The model under review builds one solid part; all positions refer to its coordinate system, in mm. Face numbers are marked on the shaded views. A direction names the side the tool comes from. Round coordinates to 2 decimals unless told otherwise and drop trailing zeros. Write each loop counter-clockwise with the first axis right and the second up, starting at its lowest first coordinate (ties: lowest second). Pieces come first, ordered by that corner, then holes. Notation, with made-up numbers: (-4, 88) -> (10, 88) arc R28 cw to (10, 126) -> close; hole circle Ø11 at (39, 4.5). An arc over 180 degrees is marked (long way). Answer as a JSON object with one key per item and string values. Group by question number.
1) Mouldability with a two-part tool opening along Z and no side actions: class the marked faces 1, 2 and 3 as pulls with the +Z half, pulls with the -Z half, needs draft (parallel to the pull), parting line crosses it, or undercut.
2) We need section D-D, the plane z = -7.75. Write out the cut boundary in (x, y), then the cut area to 3 significant figures.
3) We need section A-A, the plane x = 39.65. Write out the cut boundary in (y, z).
4) We need section B-B, the plane z = -3.5. Write out the cut boundary in (x, y), then the cut area to 3 significant figures.
5) We need section C-C, the plane y = 5.25. Write out the cut boundary in (x, z).
6) Insertion check: pin 1 Ø3.5 at (x, z) = (4.1, -7.75) entering from +Y. The pin has a flat end and moves straight along its axis. Give the tip position at first contact, or say it passes through.
7) Machinability: for the marked faces 4 and 5, which of the approach directions +Z, -Z, +X, -X, +Y, -Y give a long, thin tool a straight path to every point of the face, cutting with its end or side? Answer none if there is none.
8) To check wall thickness, follow probe 1 along X at (y, z) = (0.5, -7.75); probe 2 along X at (y, z) = (10, -11.75); probe 3 along X at (y, z) = (1.25, -3.5). State the ranges of each line that lie inside material, in increasing order. Write a range as [from, to].
from build123d import *

# Parameters (mm, degrees)
SKETCH_1_W          = 50
SKETCH_1_H          = 15.5
EXTRUDE_1_DEPTH     = 14
SKETCH_2_W          = 47
SKETCH_2_H          = 12.5
CUT_EXTRUDE_1_DEPTH = 12
SKETCH_4_R          = 1.15
SKETCH_4_R_2        = 1.806882298
SKETCH_4_W          = 23
SKETCH_4_H          = 12.5
CUT_EXTRUDE_2_DEPTH = 2


with BuildPart() as part:
    # 草图1 → 凸台-拉伸1 (new body)
    with BuildSketch(Plane(origin=(0, 0, 0), x_dir=(1, 0, 0), z_dir=(0, 1, 0))):
        with Locations((25, 7.75)):
            Rectangle(SKETCH_1_W, SKETCH_1_H)
    extrude(amount=EXTRUDE_1_DEPTH)

    # 草图2 → 切除-拉伸1 (cut)
    with BuildSketch(Plane(origin=(0, 14, 0), x_dir=(1, 0, 0), z_dir=(0, 1, 0))):
        with Locations((25, 7.75)):
            Rectangle(SKETCH_2_W, SKETCH_2_H)
    extrude(amount=-CUT_EXTRUDE_1_DEPTH, mode=Mode.SUBTRACT)

    # 草图4 → 切除-拉伸2 (cut)
    with BuildSketch(Plane(origin=(0, 2, 0), x_dir=(1, 0, 0), z_dir=(0, 1, 0))):
        with Locations(Location((4.1, 7.75, 0), (0, 0, 270))):
            Circle(SKETCH_4_R)
        with Locations(Location((31.9, 7.75, 0), (0, 0, 270))):
            Circle(SKETCH_4_R)
        with Locations(Location((39.65, 7.75, 0), (0, 0, 270))):
            Circle(SKETCH_4_R_2)
        with Locations((18, 7.75)):
            Rectangle(SKETCH_4_W, SKETCH_4_H)
    extrude(amount=-CUT_EXTRUDE_2_DEPTH, mode=Mode.SUBTRACT)


solid = part.part
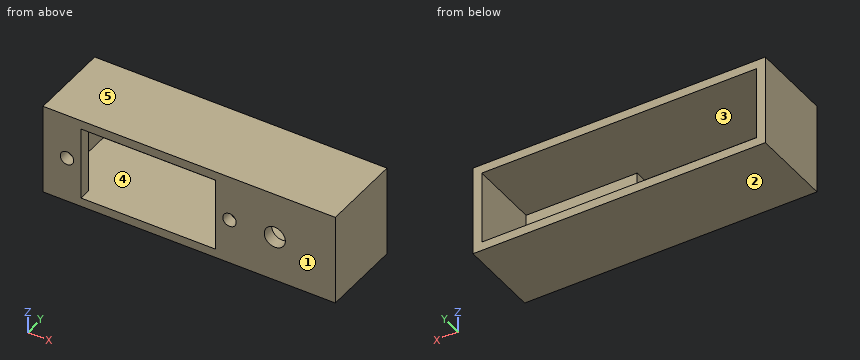
Here are the results:
{
 "1": {"face 1": "needs draft", "face 2": "pulls with the -Z half", "face 3": "undercut"},
 "2": {"outline": "(0, 0) -> (2.95, 0) -> (2.95, 2) -> (1.5, 2) -> (1.5, 14) -> (0, 14) -> close; (5.25, 0) -> (6.5, 0) -> (6.5, 2) -> (5.25, 2) -> close; (29.5, 0) -> (30.75, 0) -> (30.75, 2) -> (29.5, 2) -> close; (33.05, 0) -> (37.84, 0) -> (37.84, 2) -> (33.05, 2) -> close; (41.46, 0) -> (50, 0) -> (50, 14) -> (48.5, 14) -> (48.5, 2) -> (41.46, 2) -> close", "area": "73.6 mm^2"},
 "3": {"outline": "(0, -15.5) -> (14, -15.5) -> (14, -14) -> (2, -14) -> (2, -9.56) -> (0, -9.56) -> close; (0, -5.94) -> (2, -5.94) -> (2, -1.5) -> (14, -1.5) -> (14, 0) -> (0, 0) -> close"},
 "4": {"outline": "(0, 0) -> (6.5, 0) -> (6.5, 2) -> (1.5, 2) -> (1.5, 14) -> (0, 14) -> close; (29.5, 0) -> (50, 0) -> (50, 14) -> (48.5, 14) -> (48.5, 2) -> (29.5, 2) -> close", "area": "90.0 mm^2"},
 "5": {"outline": "(0, -15.5) -> (50, -15.5) -> (50, 0) -> (0, 0) -> close; hole (1.5, -14) -> (48.5, -14) -> (48.5, -1.5) -> (1.5, -1.5) -> close"},
 "6": {"pin 1": "stops at y = 2"},
 "7": {"face 4": "+Y", "face 5": "+Z, +X, -X, +Y, -Y"},
 "8": {"probe 1": "x = [0, 2.95], [5.25, 6.5], [29.5, 30.75], [33.05, 37.84], [41.46, 50]", "probe 2": "x = [0, 1.5], [48.5, 50]", "probe 3": "x = [0, 6.5], [29.5, 50]"}
}
